Design review of the part built by this model. Coordinates are the model's own, in mm. A direction names the side the tool comes from. Give positions to 0.01 mm unless a question says otherwise; leave off trailing zeros. Write each loop counter-clockwise with the first axis right and the second up, starting at its lowest first coordinate (ties: lowest second). Pieces come first, ordered by that corner, then holes. Notation, with made-up numbers: (17.5, -23) -> (75.5, -23) arc R21 ccw to (75.5, -14) -> close; hole circle Ø6 at (37.25, 37.25). An arc over 180 degrees is marked (long way). Answer as a JSON object with one key per item and string values.
```python
from build123d import *

# Parameters (mm, degrees)
BOSS_EXTRUDE1_DEPTH = 1.6


with BuildPart() as part:
    # Sketch2 → Boss-Extrude1 (new body)
    with BuildSketch(Plane(origin=(0, 0, 0), x_dir=(1, 0, 0), z_dir=(0, 1, 0))):
        with BuildLine():
            Line((0, 0), (12.7, 0))
            ThreePointArc((12.7, 0), (14.373884746, 4.041115254), (18.415, 5.715))
            Line((18.415, 5.715), (36.195, 5.715))
            ThreePointArc((36.195, 5.715), (40.236115254, 4.041115254), (41.91, 0))
            Line((41.91, 0), (54.61, 0))
            Line((54.61, 0), (54.61, 59.055))
            ThreePointArc((54.61, 59.055), (50.890256121, 68.035256121), (41.91, 71.755))
            Line((41.91, 71.755), (12.7, 71.755))
            ThreePointArc((12.7, 71.755), (3.719743879, 68.035256121), (0, 59.055))
            Line((0, 59.055), (0, 0))
        make_face()
    extrude(amount=BOSS_EXTRUDE1_DEPTH)


solid = part.part
```
(1) For line 1 along Z through (x, y) = (26, 1.2) (3 decimals); line 2 along X through (y, z) = (0.4, -60.5); line 3 along Z through (x, y) = (40.5, 1.25) (3 decimals), list the stretches that pass through material, from the lowest coordinate up.
Here are the results:
{"line 1": "z = -71.755 to -5.715", "line 2": "x = 0.08 to 54.53", "line 3": "z = -71.755 to -3.759"}
(2) The part is to be moulded in two halves that separate along X. For faces 1 (the cylindrical face through (50.988, 0.789, -67.936)), 2 (the flat face through (27, 1.6, -36)), 3 (the cylindrical face through (14.33, 0.789, -3.996)), say which applies: +X half, -X half, draft (parallel to the pull), parting line (faces both ways), or undercut.
Here are the results:
{"face 1": "+X half", "face 2": "draft", "face 3": "undercut"}
(3) We need section A-A, the plane y = 1.1. State the section outline as (x, z) points (3 decimals).
Here are the results:
{"outline": "(0, -59.055) arc R12.7 ccw to (12.7, -71.755) -> (41.91, -71.755) arc R12.7 ccw to (54.61, -59.055) -> (54.61, 0) -> (41.91, 0) arc R5.715 cw to (36.195, -5.715) -> (18.415, -5.715) arc R5.715 cw to (12.7, 0) -> (0, 0) -> close"}
(4) For faces 4 (the flat face through (0, 1, -30)), 5 (the flat face through (27, 1, -5.715)), list the 3-axis set-ups (+Z, -Z, +X, -X, +Y, -Y) from which the entire face can be reached by the end or side of a thin tool; tool diameter is ignored.
Here are the results:
{"face 4": "+Z, -Z, -X, +Y, -Y", "face 5": "+Z, +Y, -Y"}
(5) Clearance check with a flat-ended pin moving along its axis: pin 1 (6 mm diameter, centred on x = 17, z = -38.5, fed in from -Y). State where the tip first meets the part, or that it passes through.
Here are the results:
{"pin 1": "stops at y = 0"}
(6) We need section B-B, the plane x = 28.5. State the section outline as (y, z) points (3 decimals).
Here are the results:
{"outline": "(0, -71.755) -> (1.6, -71.755) -> (1.6, -5.715) -> (0, -5.715) -> close"}
(7) We need section C-C, the plane x = 39.5. State the section outline as (y, z) points (3 decimals), then the cut area to 3 significant figures.
Here are the results:
{"outline": "(0, -71.755) -> (1.6, -71.755) -> (1.6, -4.662) -> (0, -4.662) -> close", "area": "107 mm²"}
